Design review of the part shown in the three views and the two pictorial views. Dimensions are in mm from the part's minimum x, y and z. Round coordinates to 2 decimals unless told otherwise and drop trailing zeros. Order: outer loops, then holes, each group sorted by start corner. A loop starts at its lowest first (then second) coordinate and runs counter-clockwise, first axis right, second up.
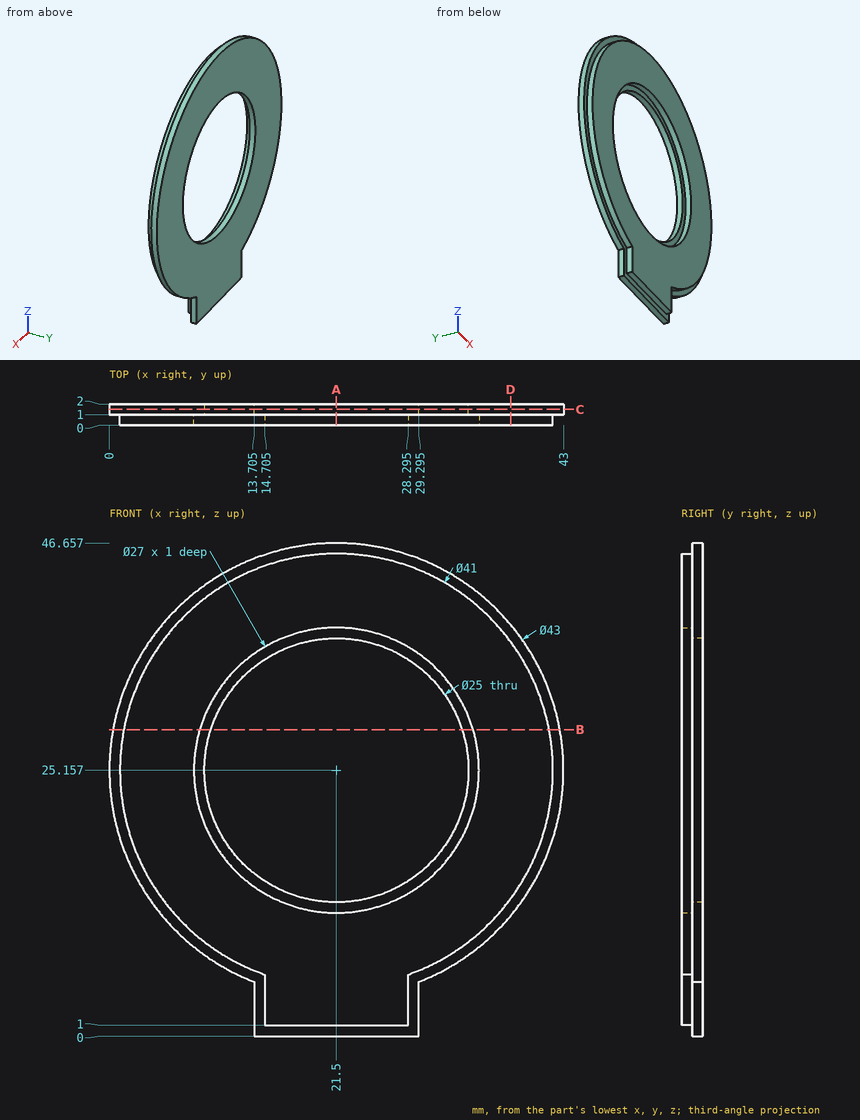
1) To check wall thickness, follow line 1 along Z through (x, y) = (21.5, 1.5); line 2 along Z through (x, y) = (21.5, 0.3); line 3 along Y through (x, z) = (9.5, 7.5). State the ranges of each line that lie inside material, in increasing order.
Results:
line 1: z = 0 to 12.66, 37.66 to 46.66
line 2: z = 1 to 11.66, 38.66 to 45.66
line 3: y = 1 to 2
2) Take a section at D-D on x = 38. Give the boundary of the cut face in (y, z).
Results:
outline: (0, 12.99) - (1, 12.99) - (1, 11.37) - (2, 11.37) - (2, 38.94) - (1, 38.94) - (1, 37.32) - (0, 37.32) - close
3) Take a section at B-B on z = 29. Give the boundary of the cut face in (x, y), plus the area to 3 significant figures.
Results:
outline: (0.35, 1) - (1.36, 1) - (1.36, 0) - (8.56, 0) - (8.56, 1) - (9.61, 1) - (9.61, 2) - (0.35, 2) - close; (33.39, 1) - (34.44, 1) - (34.44, 0) - (41.64, 0) - (41.64, 1) - (42.65, 1) - (42.65, 2) - (33.39, 2) - close
area: 32.9 mm2
4) Take a section at A-A on x = 21.5. Give the boundary of the cut face in (y, z), plus the area to 3 significant figures.
Results:
outline: (0, 1) - (1, 1) - (1, 0) - (2, 0) - (2, 12.66) - (1, 12.66) - (1, 11.66) - (0, 11.66) - close; (0, 38.66) - (1, 38.66) - (1, 37.66) - (2, 37.66) - (2, 46.66) - (1, 46.66) - (1, 45.66) - (0, 45.66) - close
area: 39.3 mm2
5) Clearance check with flat-ended pins moving along their axes: P1, Ø24.5, axis at x = 21.5, z = 25.16, coming from the +Y side; P2, Ø0.8, axis at y = 0.5, z = 4, coming from the -X side (3 decimals). State where each tip first meets the part, or that it passes through.
Results:
P1: passes through
P2: stops at x = 14.705
6) Take a section at C-C on y = 1.5. Give the boundary of the cut face in (x, z) (1 decimal), plus the area to 3 significant figures.
Results:
outline: (13.7, 0) - (29.3, 0) - (29.3, 5.1) arc R21.5 ccw (long way) to (13.7, 5.1) - close; hole circle Ø25 at (21.5, 25.2)
area: 1,030 mm2
